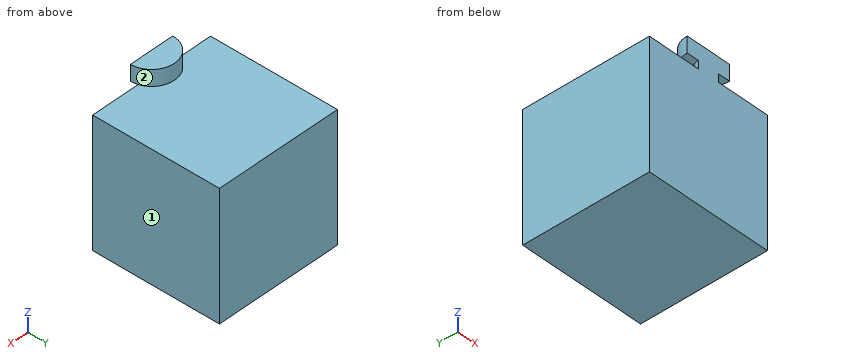
from build123d import *

# Parameters (mm, degrees)
F0_W     = 25.4
F0_H     = 25.4
F1_DEPTH = 25.4
F3_DEPTH = 1.5875
F5_DEPTH = 3.175


with BuildPart() as f1:
    # F0 (on Top) → F1 (new body)
    with BuildSketch(Plane.XY):
        Rectangle(F0_W, F0_H)
    extrude(amount=F1_DEPTH)

    # F2 (on face) → F3 (join)
    with BuildSketch(Plane.XY.offset(25.4)):
        with BuildLine():
            Line((-2.182813, -12.7), (2.182813, -12.7))
            ThreePointArc((2.182813, -12.7), (0, -10.517188), (-2.182813, -12.7))
        make_face()
    extrude(amount=F3_DEPTH)

    # F4 (on face) → F5 (join)
    with BuildSketch(Plane.XY.offset(26.9875)):
        with BuildLine():
            Line((-4.564063, -12.7), (4.564063, -12.7))
            ThreePointArc((4.564063, -12.7), (0, -8.135938), (-4.564063, -12.7))
        make_face()
    extrude(amount=F5_DEPTH)


solid = f1.part
Can you work these out from the model? Positions are in its coordinate system, mm. Face numbers are marked on the shaded views. A direction names the side the tool comes from. Give positions to 0.01 mm unless a question says otherwise; leave off trailing zeros. Order: outer loops, then holes, each group sorted by start corner. A loop starts at its lowest first (then second) coordinate and runs counter-clockwise, first axis right, second up. Notation, with made-up numbers: M -26.5,52.5 L 1.5,52.5 A23 cw 1.5,69.5 Z; hole C 42.5,61.25 d3. An arc over 180 degrees is marked long. Use a Markdown table: item, result. Add a question column.
Item 1: For the marked faces 1 and 2, which set-ups out of +Z, -Z, +X, -X, +Y, -Y let a thin tool reach every point of the face, with its end or its side?
Item 2: Suppose I cut it at B-B (x = 0). List the corners of the cut face in (y, z) for me, then the cut area to 3 significant figures.
Item 3: If I drill on L1, parallel to Z at x = -1.5, y = -10; L2, parallel to Z at x = -3, y = 10.5, over which ranges is the centre line in solid material (lowest first)? Write a range as [from, to].
Item 4: Suppose I cut it at C-C (y = -1). List the corners of the cut face in (x, z) for me.
Item 5: Will this pin go through, and if not, where does the flat tip stop? pin 1 (8 mm diameter, centred on x = 10, y = 8.5, fed in from +Z).
Item 6: Suppose I cut it at A-A (x = 2.75). List the corners of the cut face in (y, z) for me, then the cut area to 3 significant figures.
Answer sheet:
| question | item | result |
|---|---|---|
| 1 | face 1 | +Z, -Z, +X, +Y, -Y |
| 1 | face 2 | +Z, +Y |
| 2 | outline | M -12.7,0 L 12.7,0 L 12.7,25.4 L -10.52,25.4 L -10.52,26.99 L -8.14,26.99 L -8.14,30.16 L -12.7,30.16 Z |
| 2 | area | 663 mm² |
| 3 | L1 | z = [0, 25.4], [26.99, 30.16] |
| 3 | L2 | z = [0, 25.4] |
| 4 | outline | M -12.7,0 L 12.7,0 L 12.7,25.4 L -12.7,25.4 Z |
| 5 | pin 1 | stops at z = 25.4 |
| 6 | outline | M -12.7,0 L 12.7,0 L 12.7,25.4 L -12.7,25.4 Z; M -12.7,26.99 L -9.06,26.99 L -9.06,30.16 L -12.7,30.16 Z |
| 6 | area | 657 mm² |
